from build123d import *

# Parameters (mm, degrees)
MODEL_R                 = 1.5
SALIENTE_EXTRUIR1_DEPTH = 3


with BuildPart() as part:
    # Model → Saliente-Extruir1 (new body)
    with BuildSketch(Plane.XY):
        with BuildLine():
            Line((-105.943383637, 101.056539338), (-105.943383637, 47.056539338))
            ThreePointArc((-105.943383637, 47.056539338), (-104.625364152, 43.874558823), (-101.443383637, 42.556539338))
            Line((-101.443383637, 42.556539338), (-47.443383637, 42.556539338))
            ThreePointArc((-47.443383637, 42.556539338), (-45.721308191, 42.899081442), (-44.261403122, 43.874558823))
            Line((-44.261403122, 43.874558823), (-104.625364152, 104.238519853))
            ThreePointArc((-104.625364152, 104.238519853), (-105.600841533, 102.778614784), (-105.943383637, 101.056539338))
        make_face()
        with Locations((-101.443383637, 92.056539338)):
            Circle(MODEL_R, mode=Mode.SUBTRACT)
        with Locations((-101.443383637, 83.056539338)):
            Circle(MODEL_R, mode=Mode.SUBTRACT)
        with Locations((-92.443383637, 83.056539338)):
            Circle(MODEL_R, mode=Mode.SUBTRACT)
        with Locations((-101.443383637, 74.056539338)):
            Circle(MODEL_R, mode=Mode.SUBTRACT)
        with Locations((-92.443383637, 74.056539338)):
            Circle(MODEL_R, mode=Mode.SUBTRACT)
        with Locations((-83.443383637, 74.056539338)):
            Circle(MODEL_R, mode=Mode.SUBTRACT)
        with Locations((-101.443383637, 65.056539338)):
            Circle(MODEL_R, mode=Mode.SUBTRACT)
        with Locations((-92.443383637, 65.056539338)):
            Circle(MODEL_R, mode=Mode.SUBTRACT)
        with Locations((-83.443383637, 65.056539338)):
            Circle(MODEL_R, mode=Mode.SUBTRACT)
        with Locations((-74.443383637, 65.056539338)):
            Circle(MODEL_R, mode=Mode.SUBTRACT)
        with Locations((-101.443383637, 56.056539338)):
            Circle(MODEL_R, mode=Mode.SUBTRACT)
        with Locations((-92.443383637, 56.056539338)):
            Circle(MODEL_R, mode=Mode.SUBTRACT)
        with Locations((-83.443383637, 56.056539338)):
            Circle(MODEL_R, mode=Mode.SUBTRACT)
        with Locations((-74.443383637, 56.056539338)):
            Circle(MODEL_R, mode=Mode.SUBTRACT)
        with Locations((-65.443383637, 56.056539338)):
            Circle(MODEL_R, mode=Mode.SUBTRACT)
        with Locations((-101.443383637, 47.056539338)):
            Circle(MODEL_R, mode=Mode.SUBTRACT)
        with Locations((-92.443383637, 47.056539338)):
            Circle(MODEL_R, mode=Mode.SUBTRACT)
        with Locations((-83.443383637, 47.056539338)):
            Circle(MODEL_R, mode=Mode.SUBTRACT)
        with Locations((-74.443383637, 47.056539338)):
            Circle(MODEL_R, mode=Mode.SUBTRACT)
        with Locations((-65.443383637, 47.056539338)):
            Circle(MODEL_R, mode=Mode.SUBTRACT)
        with Locations((-56.443383637, 47.056539338)):
            Circle(MODEL_R, mode=Mode.SUBTRACT)
    extrude(amount=SALIENTE_EXTRUIR1_DEPTH)


solid = part.part
Work out the finished part from the listing and answer in its coordinate system (mm). Round coordinates to 2 decimals unless told otherwise and drop trailing zeros. Loops run counter-clockwise (first coordinate to the right, second up) from the corner with the lowest first, then second, coordinate; pieces in that order, holes last. Notation, with made-up numbers: M 21,-29.5 L 47,-29.5 A23 ccw 47,-7.5 Z; hole C -26.75,34 d5. An arc over 180 degrees is marked long. One line per question, with ' | ' between items. Start each with the question number.
(1) Flat-ended cylindrical pins translate along their axes: pin 1 Ø4 at (x, y) = (-65.44, 56.06) entering from -Z; pin 2 Ø1 at (x, z) = (-62.5, 1.5) entering from +Y. Find the tip coordinate at first contact, or state that the pin passes through.
(2) For a pull along X with two mould halves and no side action, classify faces 1 (the face through (-75, 42.557, 1)), 2 (the face through (-73.8, 63.7, 1.5)), 3 (the face through (-74.021, 73.634, 1.479)) as released by +X, released by -X, zero draft, split by the parting line, or undercut.
(3) A cutting plane is placed at D-D on x = -96. Write down the section's boundary in (y, z).
(4) A cutting plane is placed at A-A on x = -56. Write down the section's boundary in (y, z).
(5) Find the intervals of material crossed by line 1 (Y direction, x = -82.5, z = 1.2); line 2 (X direction, y = 83.5, z = 0.4); line 3 (Y direction, x = -66, z = 0.45), in increasing order.
(6) A cutting plane is placed at B-B on z = 0.65. Give the number of separate pieces and of enclosed holes in the cut face, plus the area to 3 significant figures.
(7) A cutting plane is placed at C-C on y = 51. Write down the section's boundary in (x, z).
Geometry check:
1) pin 1: stops at z = 0 | pin 2: stops at y = 62.61
2) face 1: zero draft | face 2: undercut | face 3: released by +X
3) outline: M 42.56,0 L 95.61,0 L 95.61,3 L 42.56,3 Z
4) outline: M 42.56,0 L 45.62,0 L 45.62,3 L 42.56,3 Z; M 48.49,0 L 55.61,0 L 55.61,3 L 48.49,3 Z
5) line 1: y = 42.56 to 45.89, 48.22 to 54.89, 57.22 to 63.89, 66.22 to 72.89, 75.22 to 82.11 | line 2: x = -105.94 to -102.88, -100.01 to -93.88, -91.01 to -83.89 | line 3: y = 42.56 to 45.66, 48.45 to 54.66, 57.45 to 65.61
6) separate pieces: 1 | enclosed holes: 21 | area: 1,830 mm²
7) outline: M -105.94,0 L -51.39,0 L -51.39,3 L -105.94,3 Z
